Source: three-view drawing plus pictorial views. Frame: mm from the lowest corner of the part. Give positions to 0.01 mm unless a question says otherwise; leave off trailing zeros. Order: outer loops, then holes, each group sorted by start corner. A loop starts at its lowest first (then second) coordinate and runs counter-clockwise, first axis right, second up. Notation, with made-up numbers: (-11, -6.5) - (47, -6.5) arc R31 cw to (47, 25.5) - close; hole circle Ø7 at (76, 71). An arc over 180 degrees is marked (long way). Answer in a Markdown table with one row per item. Add a question column.
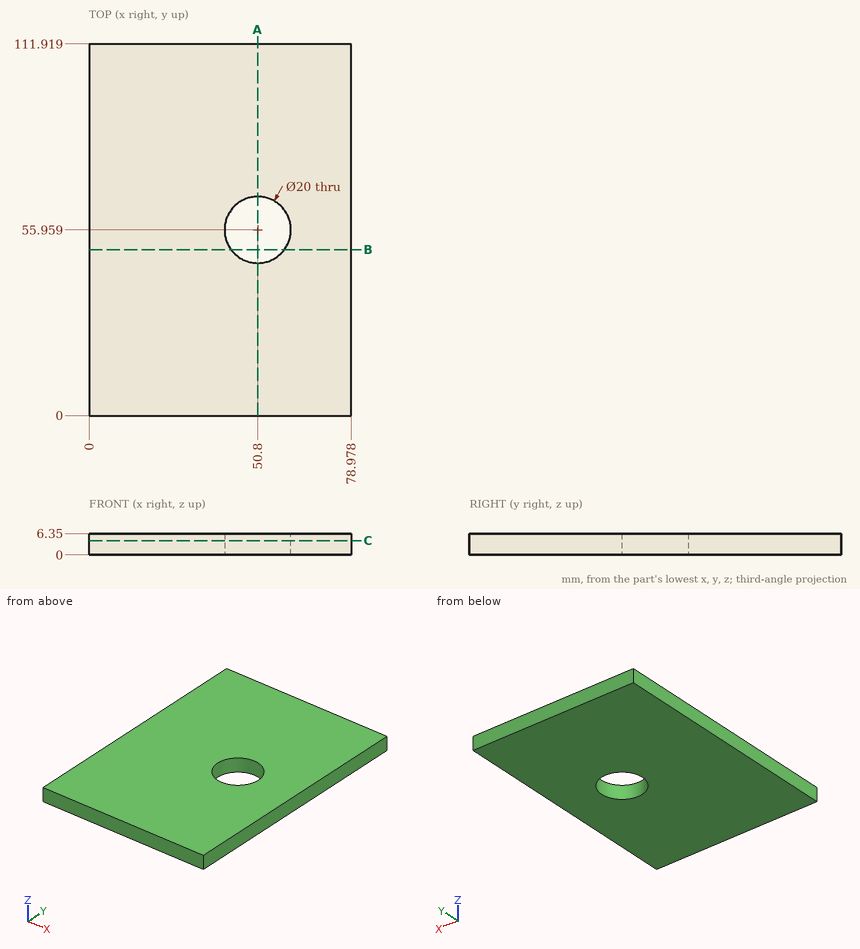
Q1. Section C-C, the plane z = 4.25. Return loops of the section in (x, y), then the cut area to 4 significant figures.
Q2. Section B-B, the plane y = 50. Return loops of the section in (x, z).
Q3. Section A-A, the plane x = 50.8. Return loops of the section in (y, z), then the cut area to 3 significant figures.
Q4. Line query: probe 1 along Y at (x, z) = (50.8, 3); probe 2 along X at (y, z) = (64, 3) (1 decimal); probe 3 along Y at (x, z) = (45, 1.75) (1 decimal). Output: solid intervals per line, ascending.
Computed:
| question | item | result |
|---|---|---|
| 1 | outline | (0, 0) - (78.98, 0) - (78.98, 111.92) - (0, 111.92) - close; hole circle Ø20 at (50.8, 55.96) |
| 1 | area | 8,525 mm^2 |
| 2 | outline | (0, 0) - (42.77, 0) - (42.77, 6.35) - (0, 6.35) - close; (58.83, 0) - (78.98, 0) - (78.98, 6.35) - (58.83, 6.35) - close |
| 3 | outline | (0, 0) - (45.96, 0) - (45.96, 6.35) - (0, 6.35) - close; (65.96, 0) - (111.92, 0) - (111.92, 6.35) - (65.96, 6.35) - close |
| 3 | area | 584 mm^2 |
| 4 | probe 1 | y = 0 to 45.96, 65.96 to 111.92 |
| 4 | probe 2 | x = 0 to 44.9, 56.7 to 79 |
| 4 | probe 3 | y = 0 to 47.8, 64.1 to 111.9 |
